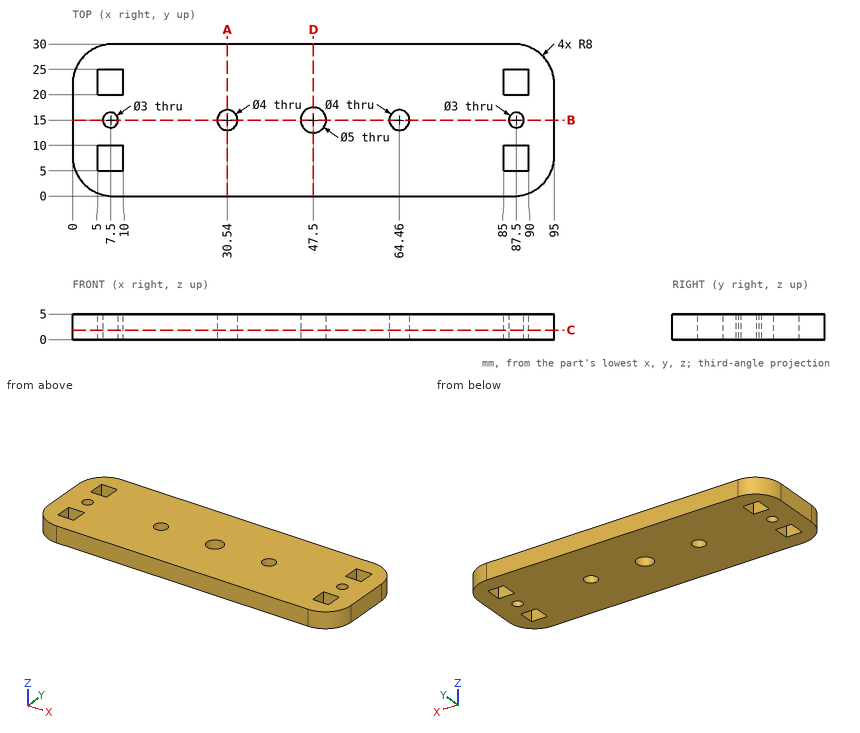
Could you check a few things on this drawing? It's one solid part, dimensions in mm from its lowest x, y, z. Give positions to 0.01 mm unless a question says otherwise; leave off trailing zeros. Order: outer loops, then holes, each group sorted by start corner. A loop starts at its lowest first (then second) coordinate and runs counter-clockwise, first axis right, second up. Notation, with made-up numbers: (75, -16) - (103, -16) arc R36 ccw to (103, 23) - close; hole circle Ø5 at (22, 76). An arc over 180 degrees is marked (long way). Answer as a JSON object with one key per item and string values. Group by question number.
Item 1: Please list where these lines run through material, in increasing order: probe 1 along Y at (x, z) = (87.5, 2.35); probe 2 along Y at (x, z) = (47.5, 1.7); probe 3 along Y at (x, z) = (64.46, 1.65).
Item 2: For P1, Ø1.5, axis at y = 6.5, z = 2.5, coming from the +X side; P2, Ø1.5, axis at x = 7, z = 3.5, coming from the +Y side, each with a flat end and sliding along its axis, tell me the tip position at first contact or that it passes through.
Item 3: If we section it at B-B on y = 15: Please give me the cut outline in (x, z), and give its area (3 significant figures).
Item 4: If we section it at D-D on x = 47.5: Please give me the cut outline in (y, z).
Item 5: If we section it at A-A on x = 30.54: Please give me the cut outline in (y, z), and give its area (3 significant figures).
Item 6: If we section it at C-C on z = 1.85: Give the number of separate pieces and of enclosed holes in the cut face, and give its area (3 significant figures).
Result set:
{
 "1": {"probe 1": "0.02 to 5, 10 to 13.5, 16.5 to 20, 25 to 29.98", "probe 2": "0 to 12.5, 17.5 to 30", "probe 3": "0 to 13, 17 to 30"},
 "2": {"P1": "x = 94.96", "P2": "y = 30"},
 "3": {"outline": "(0, 0) - (6, 0) - (6, 5) - (0, 5) - close; (9, 0) - (28.54, 0) - (28.54, 5) - (9, 5) - close; (32.54, 0) - (45, 0) - (45, 5) - (32.54, 5) - close; (50, 0) - (62.46, 0) - (62.46, 5) - (50, 5) - close; (66.46, 0) - (86, 0) - (86, 5) - (66.46, 5) - close; (89, 0) - (95, 0) - (95, 5) - (89, 5) - close", "area": "380 mm²"},
 "4": {"outline": "(0, 0) - (12.5, 0) - (12.5, 5) - (0, 5) - close; (17.5, 0) - (30, 0) - (30, 5) - (17.5, 5) - close"},
 "5": {"outline": "(0, 0) - (13, 0) - (13, 5) - (0, 5) - close; (17, 0) - (30, 0) - (30, 5) - (17, 5) - close", "area": "130 mm²"},
 "6": {"separate pieces": "1", "enclosed holes": "9", "area": "2,640 mm²"}
}
